from build123d import *

# Parameters (mm, degrees)
SKETCH_1_R          = 38
SKETCH_1_R_2        = 24.05
EXTRUDE_1_DEPTH     = 3
SKETCH_3_R          = 2
CUT_EXTRUDE_1_DEPTH = 10
CUT_EXTRUDE_2_DEPTH = 10


with BuildPart() as part:
    # 草图1 → 凸台-拉伸1 (new body)
    with BuildSketch(Plane.XY):
        Circle(SKETCH_1_R)
        Circle(SKETCH_1_R_2, mode=Mode.SUBTRACT)
    extrude(amount=EXTRUDE_1_DEPTH)

    # 草图3 → 切除-拉伸1 (cut)
    with BuildSketch(Plane.XY.offset(3)):
        with Locations((17.755280905, -21)):
            Circle(SKETCH_3_R)
        with Locations((17.755280905, 21)):
            Circle(SKETCH_3_R)
        with Locations((-17.755280905, -21)):
            Circle(SKETCH_3_R)
        with Locations((-17.755280905, 21)):
            Circle(SKETCH_3_R)
    extrude(amount=-CUT_EXTRUDE_1_DEPTH, mode=Mode.SUBTRACT)

    # 草图4 → 切除-拉伸2 (cut)
    with BuildSketch(Plane.XY.offset(3)):
        with BuildLine():
            ThreePointArc((28.095541398, -13.101166114), (31, 0), (28.095541398, 13.101166114))
            ThreePointArc((28.095541398, 13.101166114), (24.773226276, 14.310389927), (23.564002463, 10.988074805))
            ThreePointArc((23.564002463, 10.988074805), (26, 0), (23.564002463, -10.988074805))
            ThreePointArc((23.564002463, -10.988074805), (24.773226276, -14.310389927), (28.095541398, -13.101166114))
        make_face()
        with BuildLine():
            ThreePointArc((-13.101166114, -28.095541398), (0, -31), (13.101166114, -28.095541398))
            ThreePointArc((13.101166114, -28.095541398), (14.310389927, -24.773226276), (10.988074805, -23.564002463))
            ThreePointArc((10.988074805, -23.564002463), (0, -26), (-10.988074805, -23.564002463))
            ThreePointArc((-10.988074805, -23.564002463), (-14.310389927, -24.773226276), (-13.101166114, -28.095541398))
        make_face()
        with BuildLine():
            ThreePointArc((-28.095541398, 13.101166114), (-31, 0), (-28.095541398, -13.101166114))
            ThreePointArc((-28.095541398, -13.101166114), (-24.773226276, -14.310389927), (-23.564002463, -10.988074805))
            ThreePointArc((-23.564002463, -10.988074805), (-26, 0), (-23.564002463, 10.988074805))
            ThreePointArc((-23.564002463, 10.988074805), (-24.773226276, 14.310389927), (-28.095541398, 13.101166114))
        make_face()
        with BuildLine():
            ThreePointArc((13.101166114, 28.095541398), (0, 31), (-13.101166114, 28.095541398))
            ThreePointArc((-13.101166114, 28.095541398), (-14.310389927, 24.773226276), (-10.988074805, 23.564002463))
            ThreePointArc((-10.988074805, 23.564002463), (0, 26), (10.988074805, 23.564002463))
            ThreePointArc((10.988074805, 23.564002463), (14.310389927, 24.773226276), (13.101166114, 28.095541398))
        make_face()
    extrude(amount=-CUT_EXTRUDE_2_DEPTH, mode=Mode.SUBTRACT)


solid = part.part
For this review, take the finished solid that the model builds, in its own axes (mm). A direction names the side the tool comes from. Give positions to 0.01 mm unless a question says otherwise; leave off trailing zeros. Loops run counter-clockwise (first coordinate to the right, second up) from the corner with the lowest first, then second, coordinate; pieces in that order, holes last.
Item 1: Take a section at D-D, the plane x = 27. State the section outline as (y, z) points, and give its area (3 significant figures).
Item 2: Tool access review of faces 1 (the cylindrical face through (0, -31, 2)), 2 (the flat face through (25, 1, 0)): name each direction out of +Z, -Z, +X, -X, +Y, -Y from which nothing blocks a thin tool from reaching the whole face with its end or side.
Item 3: Take a section at C-C, the plane z = 0.45. Give the number of separate pieces and of enclosed holes in the cut face, and give its area (3 significant figures).
Item 4: Insertion check: pin 1 (4.5 mm diameter, centred on x = -17.76, y = -21, fed in from +Z); pin 2 (1 mm diameter, centred on y = 26.5, z = 2.5, fed in from +X). Each pin has a flat end and moves straight along its axis. Give the tip position at first contact, or say it passes through.
Item 5: For line 1 along Y through (x, z) = (-0.5, 1.95); line 2 along Y through (x, z) = (4.5, 1); line 3 along X through (y, z) = (-20, 1.4), list the stretches that pass through material, from the lowest coordinate up.
Item 6: Take a section at A-A, the plane x = 0. State the section outline as (y, z) points, and give its area (3 significant figures).
Item 7: Draft analysis for pull direction Y (two halves, no side actions). For faces 3 (the cylindrical face through (-24.82, -14.33, 1.52)), 4 (the flat face through (25, 1, 3)), 5 (the cylindrical face through (17.535, -33.713, 1.479)), state which applies: +Y half, -Y half, draft (parallel to the pull), parting line (faces both ways), or undercut.
Calculated:
1. outline: (-26.74, 0) - (-14.25, 0) - (-14.25, 3) - (-26.74, 3) - close; (14.25, 0) - (26.74, 0) - (26.74, 3) - (14.25, 3) - close
1. area: 74.9 mm2
2. face 1: +Z, -Z
2. face 2: -Z, +X, -X, +Y, -Y
3. separate pieces: 1
3. enclosed holes: 9
3. area: 2,090 mm2
4. pin 1: stops at z = 3
4. pin 2: stops at x = 27.71
5. line 1: y = -38 to -31, -26 to -24.04, 24.04 to 26, 31 to 38
5. line 2: y = -37.73 to -30.67, -25.61 to -23.63, 23.63 to 25.61, 30.67 to 37.73
5. line 3: x = -32.31 to -19.49, -16.02 to -13.36, 13.36 to 16.02, 19.49 to 32.31
6. outline: (-38, 0) - (-31, 0) - (-31, 3) - (-38, 3) - close; (-26, 0) - (-24.05, 0) - (-24.05, 3) - (-26, 3) - close; (24.05, 0) - (26, 0) - (26, 3) - (24.05, 3) - close; (31, 0) - (38, 0) - (38, 3) - (31, 3) - close
6. area: 53.7 mm2
7. face 3: undercut
7. face 4: draft
7. face 5: parting line
